Geometry: final body of the model. Coordinates: model frame, mm. Round coordinates to 2 decimals unless told otherwise and drop trailing zeros. Write each loop counter-clockwise with the first axis right and the second up, starting at its lowest first coordinate (ties: lowest second). Pieces come first, ordered by that corner, then holes. Notation, with made-up numbers: (23, 7) - (79, 7) arc R22 ccw to (79, 23) - close; hole circle Ø5 at (84.25, -17.75). An arc over 180 degrees is marked (long way). Write each question's results on one line, items separated by ' | '.
Autodesk Inventor part; units mm, degrees
ref_plane "YZ Plane" through (0, 0, 0) normal (1, 0, 0) x (0, 1, 0)
ref_plane "XZ Plane" through (0, 0, 0) normal (0, 1, 0) x (-1, 0, 0)
ref_plane "XY Plane" through (0, 0, 0) normal (0, 0, 1) x (1, 0, 0)
sketch "草图1" plane through (0, 0, 0) normal (0, 0, 1) x (1, 0, 0)
  line L0 (-48, 0) -> (48, 0) construction
  line L1 (-48, -5) -> (48, -5)
  line L2 (48, 5) -> (-48, 5)
  arc A0 (-48, 5) -> (-48, -5) centre (-48, 0) ccw
  arc A1 (48, -5) -> (48, 5) centre (48, 0) ccw
  point P0 (0, 0)
  dimension "d1" = 96
  dimension "d4" = 10
extrude "拉伸1" add sketch "草图1" along normal blind 3
sketch "草图2" plane through (0, 0, 0) normal (0, 0, -1) x (-1, 0, 0)
  arc A0 (48, -5) -> (48, 5) centre (48, 0) ccw
  circle A1 centre (48, 0) radius 2
  line L0 (0, 0) -> (0, -18.0747)
  arc A2 (-48, 5) -> (-48, -5) centre (-48, 0) ccw
  circle A3 centre (-48, 0) radius 2
  dimension "d5" = 4
extrude "拉伸2" cut sketch "草图2" against normal blind 10
properties part number "连杆1"
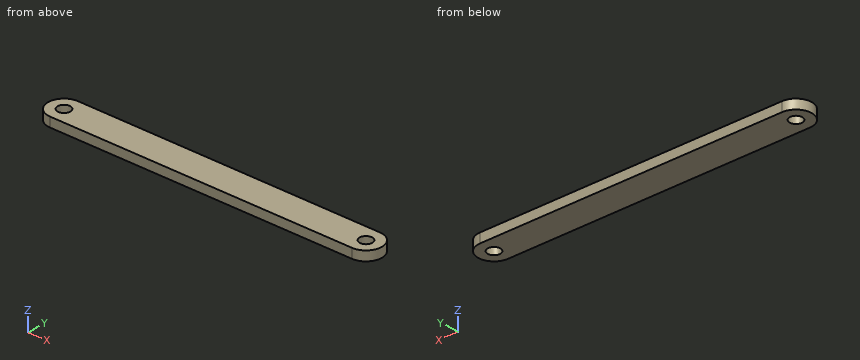
Q1. Section query A-A, the plane y = 0. Return loops of the section in (x, z).
Answer block:
outline: (-53, 0) - (-50, 0) - (-50, 3) - (-53, 3) - close; (-46, 0) - (46, 0) - (46, 3) - (-46, 3) - close; (50, 0) - (53, 0) - (53, 3) - (50, 3) - close
Q2. Ray query, line 1 along Y through (x, z) = (48, 0.6); line 2 along X through (y, z) = (0.5, 1.95); line 3 along X through (y, z) = (1, 2.8). Return the intervals inside material, ascending.
Answer block:
line 1: -5 to -2, 2 to 5 | line 2: -52.97 to -49.94, -46.06 to 46.06, 49.94 to 52.97 | line 3: -52.9 to -49.73, -46.27 to 46.27, 49.73 to 52.9
Q3. Section query B-B, the plane z = 0.55. Return loops of the section in (x, y).
Answer block:
outline: (-48, -5) - (48, -5) arc R5 ccw to (48, 5) - (-48, 5) arc R5 ccw to start; hole circle Ø4 at (-48, 0); hole circle Ø4 at (48, 0)
